CAD build for the part. Positions are in the model's coordinates, mm. Face numbers are marked on the shaded views. A direction names the side the tool comes from. Coordinates: 2 decimals unless noted, no trailing zeros. Order: outer loops, then holes, each group sorted by start corner. A loop starts at its lowest first (then second) coordinate and runs counter-clockwise, first axis right, second up. Notation, with made-up numbers: (-12.5, 70) - (-3.5, 70) arc R23 ccw to (-3.5, 101) - close; hole circle Ø5 at (-6.75, 73). An arc over 180 degrees is marked (long way). Return JSON: item names as keys, results as strings.
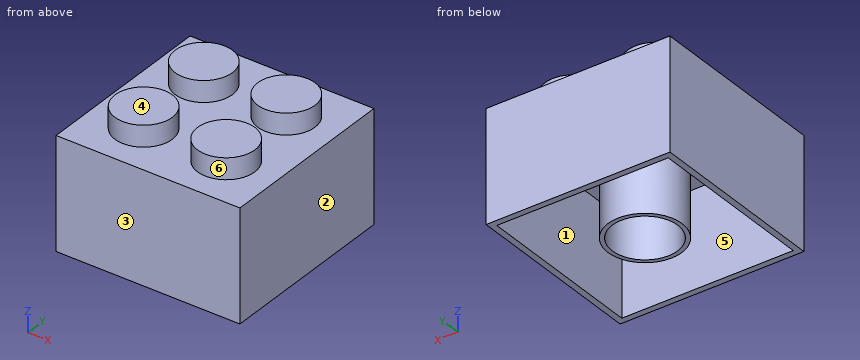
from build123d import *

# Parameters (mm, degrees)
F0_W     = 15.494
F0_H     = 15.494
F1_DEPTH = 9.398
F2_R     = 2.413
F3_DEPTH = 1.778
F4_W     = 14.4526
F4_H     = 14.4526
F5_DEPTH = 8.128
F6_R     = 3.1115
F7_DEPTH = 8.128
F8_R     = 2.7559
F9_DEPTH = 8.128


with BuildPart() as f1:
    # F0 (on Top) → F1 (new body)
    with BuildSketch(Plane.XY):
        Rectangle(F0_W, F0_H)
    extrude(amount=F1_DEPTH)

    # F2 (on face) → F3 (join)
    with BuildSketch(Plane.XY.offset(9.398)):
        with Locations((-3.4798, 3.4798)):
            Circle(F2_R)
        with Locations((3.4798, 3.4798)):
            Circle(F2_R)
        with Locations((3.4798, -3.4798)):
            Circle(F2_R)
        with Locations((-3.4798, -3.4798)):
            Circle(F2_R)
    extrude(amount=F3_DEPTH)

    # F4 (on face) → F5 (cut)
    with BuildSketch(Plane(origin=(0, 0, 0), x_dir=(1, 0, 0), z_dir=(0, 0, -1))):
        Rectangle(F4_W, F4_H)
    extrude(amount=-F5_DEPTH, mode=Mode.SUBTRACT)

    # F6 (on face) → F7 (join)
    with BuildSketch(Plane(origin=(0, 0, 8.128), x_dir=(1, 0, 0), z_dir=(0, 0, -1))):
        Circle(F6_R)
    extrude(amount=F7_DEPTH)

    # F8 (on face) → F9 (cut)
    with BuildSketch(Plane(origin=(0, 0, 0), x_dir=(1, 0, 0), z_dir=(0, 0, -1))):
        Circle(F8_R)
    extrude(amount=-F9_DEPTH, mode=Mode.SUBTRACT)


solid = f1.part
Item 1: Mould opens along Y. For the marked faces 1, 2 and 3 say: released by +Y, released by -Y, zero draft, split by the parting line, or undercut.
Findings below:
{"face 1": "undercut", "face 2": "zero draft", "face 3": "released by -Y"}
Item 2: Which spindle directions (+Z, -Z, +X, -X, +Y, -Y) get a long thin tool onto all of the face, cutting with end or side? Do the marked faces 4, 5 and 6. Say none if no direction does.
Findings below:
{"face 4": "+Z, +X, -X, +Y, -Y", "face 5": "-Z", "face 6": "+Z"}
Item 3: Wall check: L1, parallel to Y at x = 0, z = 5; L2, parallel to X at y = -7, z = 5.75. Give the ranges that are in metal, low to high. Write a range as [from, to].
Findings below:
{"L1": "y = [-7.75, -7.23], [-3.11, -2.76], [2.76, 3.11], [7.23, 7.75]", "L2": "x = [-7.75, -7.23], [7.23, 7.75]"}
Item 4: Band-saw the part on C-C, the plane x = 6.5. List the corners of the cut face in (y, z), then the cut area to 3 significant figures.
Findings below:
{"outline": "(-7.75, 0) - (-7.23, 0) - (-7.23, 8.13) - (7.23, 8.13) - (7.23, 0) - (7.75, 0) - (7.75, 9.4) - (-7.75, 9.4) - close", "area": "28.1 mm²"}
Item 5: Band-saw the part on A-A, the plane z = 2. List the corners of the cut face in (x, y), then the cut area to 3 significant figures.
Findings below:
{"outline": "(-7.75, -7.75) - (7.75, -7.75) - (7.75, 7.75) - (-7.75, 7.75) - close; circle Ø6.22 at (0, 0); hole (-7.23, -7.23) - (7.23, -7.23) - (7.23, 7.23) - (-7.23, 7.23) - close; hole circle Ø5.51 at (0, 0)", "area": "37.7 mm²"}
Item 6: Band-saw the part on B-B, the plane y = 0. List the corners of the cut face in (x, z), then the cut area to 3 significant figures.
Findings below:
{"outline": "(-7.75, 0) - (-7.23, 0) - (-7.23, 8.13) - (-3.11, 8.13) - (-3.11, 0) - (-2.76, 0) - (-2.76, 8.13) - (2.76, 8.13) - (2.76, 0) - (3.11, 0) - (3.11, 8.13) - (7.23, 8.13) - (7.23, 0) - (7.75, 0) - (7.75, 9.4) - (-7.75, 9.4) - close", "area": "33.9 mm²"}
